```python
from build123d import *

# Parameters (mm, degrees)
SKETCH1_W           = 457.2
SKETCH1_H           = 304.8
SKETCH1_R           = 25.4
CHAMBER_BASE_DEPTH  = 6.35
SKETCH2_W           = 457.2
SKETCH2_H           = 304.8
BACK_WALL_DEPTH     = 6.35
SKETCH3_W           = 463.55
SKETCH3_H           = 457.2
SIDE_WALL_2_DEPTH   = 6.35
SKETCH5_W           = 463.55
SKETCH5_H           = 457.2
SIDE_WALL_3_DEPTH   = 6.35
SKETCH6_W           = 457.2
SKETCH6_H           = 317.5
BOSS_EXTRUDE1_DEPTH = 6.35


with BuildPart() as part:
    # Sketch1 → Chamber Base (new body)
    with BuildSketch(Plane.XY):
        with Locations((228.6, 152.4)):
            Rectangle(SKETCH1_W, SKETCH1_H)
        with Locations((228.6, 152.4)):
            Circle(SKETCH1_R, mode=Mode.SUBTRACT)
    extrude(amount=CHAMBER_BASE_DEPTH)

    # Sketch2 → Back wall (add)
    with BuildSketch(Plane(origin=(457.2, 0, 0), x_dir=(0, 0, -1), z_dir=(1, 0, 0))):
        with Locations((-228.6, 152.4)):
            Rectangle(SKETCH2_W, SKETCH2_H)
    extrude(amount=BACK_WALL_DEPTH)

    # Sketch3 → Side wall 2 (add)
    with BuildSketch(Plane(origin=(0, 304.8, 0), x_dir=(1, 0, 0), z_dir=(0, 1, 0))):
        with Locations((231.775, -228.6)):
            Rectangle(SKETCH3_W, SKETCH3_H)
    extrude(amount=SIDE_WALL_2_DEPTH)

    # Sketch5 → Side wall 3 (add)
    with BuildSketch(Plane.XZ):
        with Locations((231.775, 228.6)):
            Rectangle(SKETCH5_W, SKETCH5_H)
    extrude(amount=SIDE_WALL_3_DEPTH)

    # Sketch6 → Boss-Extrude1 (add)
    with BuildSketch(Plane.ZY):
        with Locations((228.6, 152.4)):
            Rectangle(SKETCH6_W, SKETCH6_H)
    extrude(amount=BOSS_EXTRUDE1_DEPTH)


solid = part.part
```
Geometry: final body of the model. Coordinates: model frame, mm. A direction names the side the tool comes from. Coordinates: 2 decimals unless noted, no trailing zeros. Order: outer loops, then holes, each group sorted by start corner. A loop starts at its lowest first (then second) coordinate and runs counter-clockwise, first axis right, second up. Notation, with made-up numbers: (32, -28) - (36, -28) arc R26 ccw to (36, 8) - close; hole circle Ø1 at (80, -33.75). An arc over 180 degrees is marked (long way). Return JSON: item names as keys, results as strings. Group by question number.
1. Cut plane B-B (x = 228.6). Output: boundary loops of the cut face in (y, z), plus the area to 3 significant figures.
2. Pull-direction query (Y, two-part tool) for faces 3 (the face through (463.55, 155, 225)), 4 (the face through (225, 304.8, 229)), 5 (the face through (232, 311.15, 225)); classes: pulls with the +Y half, pulls with the -Y half, needs draft (parallel to the pull), parting line crosses it, or undercut.
3. Cut plane A-A (y = 152.4). Output: boundary loops of the cut face in (x, z), plus the area to 3 significant figures.
4. Set-up query: faces 1 (the face through (-6.35, 155, 225)), 2 (the face through (457.2, 155, 235)). Return all of +Z, -Z, +X, -X, +Y, -Y with unobstructed straight access to the full face (end or side cutting, diameter ignored); none if empty.
5. Material intervals for line 1 along X through (y, z) = (50, 320.5); line 2 along X through (y, z) = (152, 1); line 3 along Y through (x, z) = (238.5, 195.5), sorted ascending. Write a range as [from, to].
6. Cut plane D-D (x = 72). Output: boundary loops of the cut face in (y, z).
7. Pin query (flat end, axial travel): pin 1 (1.5 mm diameter, centred on x = 136.5, y = 34, fed in from +Z); pin 2 (8 mm diameter, centred on x = 109, y = 181, fed in from -Z). Return the tip coordinate at first contact, or that it passes through.
8. Cut plane C-C (z = 380). Output: boundary loops of the cut face in (x, y).
Resolved:
{
 "1": {"outline": "(-6.35, 0) - (127, 0) - (127, 6.35) - (0, 6.35) - (0, 457.2) - (-6.35, 457.2) - close; (177.8, 0) - (311.15, 0) - (311.15, 457.2) - (304.8, 457.2) - (304.8, 6.35) - (177.8, 6.35) - close", "area": "7,420 mm²"},
 "2": {"face 3": "needs draft", "face 4": "undercut", "face 5": "pulls with the +Y half"},
 "3": {"outline": "(-6.35, 0) - (203.2, 0) - (203.2, 6.35) - (0, 6.35) - (0, 457.2) - (-6.35, 457.2) - close; (254, 0) - (463.55, 0) - (463.55, 457.2) - (457.2, 457.2) - (457.2, 6.35) - (254, 6.35) - close", "area": "8,390 mm²"},
 "4": {"face 1": "+Z, -Z, -X, +Y, -Y", "face 2": "+Z"},
 "5": {"line 1": "x = [-6.35, 0], [457.2, 463.55]", "line 2": "x = [-6.35, 203.2], [254, 463.55]", "line 3": "y = [-6.35, 0], [304.8, 311.15]"},
 "6": {"outline": "(-6.35, 0) - (311.15, 0) - (311.15, 457.2) - (304.8, 457.2) - (304.8, 6.35) - (0, 6.35) - (0, 457.2) - (-6.35, 457.2) - close"},
 "7": {"pin 1": "stops at z = 6.35", "pin 2": "stops at z = 0"},
 "8": {"outline": "(-6.35, -6.35) - (463.55, -6.35) - (463.55, 311.15) - (-6.35, 311.15) - close; hole (0, 0) - (457.2, 0) - (457.2, 304.8) - (0, 304.8) - close"}
}
